from build123d import *

# Parameters (mm, degrees)
SALIENTE_EXTRUIR1_DEPTH = 55
CROQUIS2_R              = 9.525
CORTAR_EXTRUIR1_DEPTH   = 3.025
CROQUIS3_W              = 4.95
CROQUIS3_H              = 34.95
SALIENTE_EXTRUIR2_DEPTH = 10
REDONDEO1_R             = 8
CORTAR_EXTRUIR2_DEPTH   = 8


with BuildPart() as part:
    # Croquis1 → Saliente-Extruir1 (new body)
    with BuildSketch(Plane.XY):
        with BuildLine():
            Line((-40, 0), (-5, 0))
            ThreePointArc((-5, 0), (0, 5), (5, 0))
            Line((5, 0), (40, 0))
            Line((40, 0), (40, 22))
            Line((40, 22), (-40, 22))
            Line((-40, 22), (-40, 0))
        make_face()
    extrude(amount=SALIENTE_EXTRUIR1_DEPTH)

    # Croquis2 → Cortar-Extruir1 (cut, symmetric)
    with BuildSketch(Plane.XY.offset(27.5)):
        Circle(CROQUIS2_R)
    extrude(amount=CORTAR_EXTRUIR1_DEPTH, both=True, mode=Mode.SUBTRACT)

    # Croquis3 → Saliente-Extruir2 (add)
    with BuildSketch(Plane.XZ):
        with Locations((-32.525, 27.5)):
            Rectangle(CROQUIS3_W, CROQUIS3_H)
        with Locations((32.525, 27.5)):
            Rectangle(CROQUIS3_W, CROQUIS3_H)
    extrude(amount=SALIENTE_EXTRUIR2_DEPTH)

    # Redondeo1
    redondeo1_edges = [part.edges().sort_by_distance(p)[0] for p in [
        (40, 11, 55),
        (-40, 11, 55),
        (-40, 11, 0),
        (40, 11, 0),
    ]]
    fillet(redondeo1_edges, radius=REDONDEO1_R)

    # Croquis6 → Cortar-Extruir2 (cut)
    with BuildSketch(Plane(origin=(0, 22, 0), x_dir=(1, 0, 0), z_dir=(0, 1, 0))):
        Polygon((-23.75, -45.25), (-2.5, -45.25), (-2.5, -47.75), (2.5, -47.75), (2.5, -45.25), (23.75, -45.25), (23.75, -9.75), (-23.75, -9.75), (-23.75, -25), (-26.25, -25), (-26.25, -30), (-23.75, -30), align=None)
    extrude(amount=-CORTAR_EXTRUIR2_DEPTH, mode=Mode.SUBTRACT)


solid = part.part
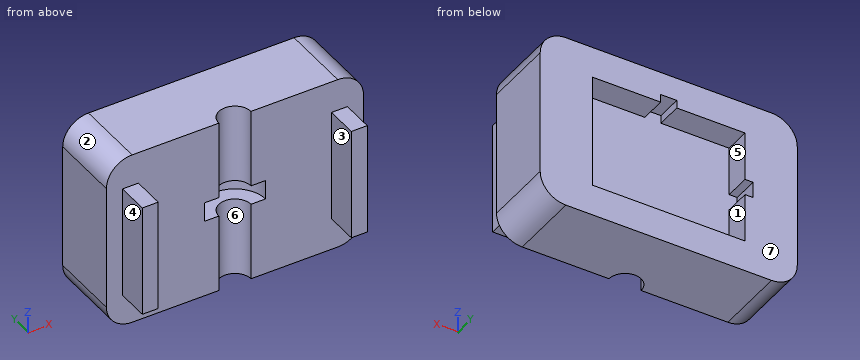
Can you work these out from the model? Positions are in its coordinate system, mm. Face numbers are marked on the shaded views. A direction names the side the tool comes from. Coordinates: 2 decimals unless noted, no trailing zeros. Order: outer loops, then holes, each group sorted by start corner. A loop starts at its lowest first (then second) coordinate and runs counter-clockwise, first axis right, second up. Notation, with made-up numbers: (38, 60) -> (78, 60) arc R27 ccw to (78, 80) -> close; hole circle Ø3 at (49.5, 57). An arc over 180 degrees is marked (long way). Use one line per item in the form item = value.
Q1. Imagine slicing it at B-B, the plane x = 20. List the corners of the cut face in (y, z) for me, then the cut area to 3 significant figures.
From the geometry:
outline = (0, 0) -> (22, 0) -> (22, 9.75) -> (14, 9.75) -> (14, 45.25) -> (22, 45.25) -> (22, 55) -> (0, 55) -> close
area = 926 mm²
Q2. We'd pull the mould along X, two halves only. Please class the marked faces 4, 5, 6 and 7: released by +X, released by -X, zero draft, split by the parting line, or undercut.
From the geometry:
face_4 = released by -X
face_5 = undercut
face_6 = undercut
face_7 = zero draft
Q3. Imagine slicing it at D-D, the plane y = -2. List the corners of the cut face in (x, z) for me (3 decimals), then the cut area to 3 significant figures.
From the geometry:
outline = (-35, 10.025) -> (-30.05, 10.025) -> (-30.05, 44.975) -> (-35, 44.975) -> close; (30.05, 10.025) -> (35, 10.025) -> (35, 44.975) -> (30.05, 44.975) -> close
area = 346 mm²
Q4. Which directions (+Z, -Z, +X, -X, +Y, -Y) give clear straight access to the entire face, cutting with the end or side of a thin tool? Please do the marked faces 1, 2 and 3.
From the geometry:
face_1 = +Y
face_2 = +Z, -X, +Y, -Y
face_3 = +Z, -Z, -Y
Q5. Will these pins go through, and if not, where does the flat tip stop? P1, Ø4, axis at x = 5, z = 11, coming from the -Y side; P2, Ø2.5, axis at x = 32.5, y = -5.5, coming from the +Z side (3 decimals); P3, Ø3, axis at y = -4, z = 20, coming from the +X side.
From the geometry:
P1 = 0
P2 = 44.975
P3 = 35
Q6. Imagine slicing it at C-C, the plane z = 28. List the corners of the cut face in (x, y) for me (3 decimals), then the cut area to 3 significant figures.
From the geometry:
outline = (-40, 0) -> (-35, 0) -> (-35, -10) -> (-30.05, -10) -> (-30.05, 0) -> (-9.525, 0) arc R9.525 cw to (9.525, 0) -> (30.05, 0) -> (30.05, -10) -> (35, -10) -> (35, 0) -> (40, 0) -> (40, 22) -> (23.75, 22) -> (23.75, 14) -> (-26.25, 14) -> (-26.25, 22) -> (-40, 22) -> close
area = 1,320 mm²
Q7. I need wall thicknesses on L1, parallel to X at y = -6, z = 39; L2, parallel to X at y = 17, z = 29; L3, parallel to Z at x = 8, y = 19.5. Which ranges of each line are inside material? Lowest first, please.
From the geometry:
L1 = -35 to -30.05, 30.05 to 35
L2 = -40 to -26.25, 23.75 to 40
L3 = 0 to 9.75, 45.25 to 55
Q8. Imagine slicing it at A-A, the plane y = 20. List the corners of the cut face in (x, z) for me.
From the geometry:
outline = (-40, 8) arc R8 ccw to (-32, 0) -> (32, 0) arc R8 ccw to (40, 8) -> (40, 47) arc R8 ccw to (32, 55) -> (-32, 55) arc R8 ccw to (-40, 47) -> close; hole (-26.25, 25) -> (-23.75, 25) -> (-23.75, 9.75) -> (23.75, 9.75) -> (23.75, 45.25) -> (2.5, 45.25) -> (2.5, 47.75) -> (-2.5, 47.75) -> (-2.5, 45.25) -> (-23.75, 45.25) -> (-23.75, 30) -> (-26.25, 30) -> close
